```python
from build123d import *

# Parameters (mm, degrees)
SKETCH3_R           = 1.9
SKETCH3_R_2         = 11.5
BOSS_EXTRUDE2_DEPTH = 5


with BuildPart() as part:
    # Sketch3 → Boss-Extrude2 (new body)
    with BuildSketch(Plane.XY):
        with BuildLine():
            Line((-50, 45), (50, 45))
            ThreePointArc((50, 45), (57.071067812, 42.071067812), (60, 35))
            Line((60, 35), (60, -35))
            ThreePointArc((60, -35), (57.071067812, -42.071067812), (50, -45))
            Line((50, -45), (-50, -45))
            ThreePointArc((-50, -45), (-57.071067812, -42.071067812), (-60, -35))
            Line((-60, -35), (-60, 35))
            ThreePointArc((-60, 35), (-57.071067812, 42.071067812), (-50, 45))
        make_face()
        with Locations((-50, 35)):
            Circle(SKETCH3_R, mode=Mode.SUBTRACT)
        with Locations((50, 35)):
            Circle(SKETCH3_R, mode=Mode.SUBTRACT)
        with Locations((50, -35)):
            Circle(SKETCH3_R, mode=Mode.SUBTRACT)
        with Locations((-50, -35)):
            Circle(SKETCH3_R, mode=Mode.SUBTRACT)
        Circle(SKETCH3_R_2, mode=Mode.SUBTRACT)
    extrude(amount=BOSS_EXTRUDE2_DEPTH)


solid = part.part
```
The listing builds one solid part. Answer for the finished solid, in the listing's coordinates (mm). Give positions to 0.01 mm unless a question says otherwise; leave off trailing zeros. Order: outer loops, then holes, each group sorted by start corner. A loop starts at its lowest first (then second) coordinate and runs counter-clockwise, first axis right, second up. Notation, with made-up numbers: (-18.75, -2) -> (-3.75, -2) arc R24 cw to (-3.75, 33) -> close; hole circle Ø4 at (-8, 45.25). An arc over 180 degrees is marked (long way). Answer as CSV lines item,"result". Start each with the question number.
Q1. A cutting plane is placed at B-B (y = 0). Determine the outline of the cut face in (x, z).
Q2. Find the intervals of material crossed by L1, parallel to Y at x = 50, z = 3.7; L2, parallel to Y at x = 0, z = 2.4; L3, parallel to X at y = 9, z = 1.1, in increasing order.
Q3. A cutting plane is placed at C-C (z = 3.1). Determine the outline of the cut face in (x, y).
Q4. Given pin 1 (2.5 mm diameter, centred on x = 50, y = -35, fed in from +Z), flat-ended and moving along its own axis, determine where the tip first touches the part or whether it passes through.
Q5. A cutting plane is placed at A-A (x = 0). Determine the outline of the cut face in (y, z), then the cut area to 3 significant figures.
Results found:
1,outline,"(-60, 0) -> (-11.5, 0) -> (-11.5, 5) -> (-60, 5) -> close; (11.5, 0) -> (60, 0) -> (60, 5) -> (11.5, 5) -> close"
2,L1,"-45 to -36.9, -33.1 to 33.1, 36.9 to 45"
2,L2,"-45 to -11.5, 11.5 to 45"
2,L3,"-60 to -7.16, 7.16 to 60"
3,outline,"(-60, -35) arc R10 ccw to (-50, -45) -> (50, -45) arc R10 ccw to (60, -35) -> (60, 35) arc R10 ccw to (50, 45) -> (-50, 45) arc R10 ccw to (-60, 35) -> close; hole circle Ø3.8 at (-50, -35); hole circle Ø3.8 at (-50, 35); hole circle Ø23 at (0, 0); hole circle Ø3.8 at (50, -35); hole circle Ø3.8 at (50, 35)"
4,pin 1,"through"
5,outline,"(-45, 0) -> (-11.5, 0) -> (-11.5, 5) -> (-45, 5) -> close; (11.5, 0) -> (45, 0) -> (45, 5) -> (11.5, 5) -> close"
5,area,"335 mm2"
